```python
from build123d import *

# Parameters (mm, degrees)
F0_W     = 100
F0_H     = 270
F1_DEPTH = 100
F2_SIZE  = 75
F3_SIZE  = 5
F4_R     = 5


with BuildPart() as f1:
    # F0 (on Top) → F1 (new body)
    with BuildSketch(Plane.XY):
        Rectangle(F0_W, F0_H)
    extrude(amount=F1_DEPTH)

    # F2
    f2_edges = [f1.edges().sort_by_distance(p)[0] for p in [
        (0, -135, 0),
        (0, 135, 0),
    ]]
    chamfer(f2_edges, length=F2_SIZE)

    # F3
    f3_edges = [f1.edges().sort_by_distance(p)[0] for p in [
        (0, -135, 75),
        (0, 135, 75),
    ]]
    chamfer(f3_edges, length=F3_SIZE)

    # F4
    f4_edges = [f1.edges().sort_by_distance(p)[0] for p in [
        (0, 135, 80),
        (0, 131.464466, 71.464466),
        (0, -135, 80),
        (0, -131.464466, 71.464466),
    ]]
    fillet(f4_edges, radius=F4_R)


solid = f1.part
```
Design review of the part built by this model. Coordinates are the model's own, in mm. Give positions to 0.01 mm unless a question says otherwise; leave off trailing zeros. Loops run counter-clockwise (first coordinate to the right, second up) from the corner with the lowest first, then second, coordinate; pieces in that order, holes last. Notation, with made-up numbers: M -28.5,-25 L -17.5,-25 A36 cw -17.5,9 Z; hole C 64.5,41.25 d1. An arc over 180 degrees is marked long. Return JSON: item names as keys, results as strings. Group by question number.
Item 1: For probe 1 along Y at (x, z) = (-15, 22); probe 2 along Y at (x, z) = (-25.5, 39); probe 3 along Z at (x, y) = (5, -99.5), list the stretches that pass through material, from the lowest coordinate up.
Item 2: We need section A-A (x = 25). Give the boundary of the cut face in (y, z), and give its area (3 significant figures).
Item 3: We need section B-B (y = 108). Give the boundary of the cut face in (x, z).
Item 4: Insertion check: pin 1 Ø5 at (x, z) = (-34.5, 10) entering from +Y; pin 2 Ø4 at (x, z) = (-24.5, 16) entering from -Y; pin 3 Ø12 at (x, z) = (-12.5, 26.5) entering from -Y. Each pin has a flat end and moves straight along its axis. Give the tip position at first contact, or say it passes through.
Item 5: We need section C-C (z = 16). Give the boundary of the cut face in (x, y).
Output:
{
 "1": {"probe 1": "y = -82 to 82", "probe 2": "y = -99 to 99", "probe 3": "z = 39.5 to 100"},
 "2": {"outline": "M -135,80.99 A5 ccw -134.62,79.08 L -131.85,72.38 A5 ccw -130.76,70.76 L -60,0 L 60,0 L 130.76,70.76 A5 ccw 131.85,72.38 L 134.62,79.08 A5 ccw 135,80.99 L 135,100 L -135,100 Z", "area": "21,400 mm^2"},
 "3": {"outline": "M -50,48 L 50,48 L 50,100 L -50,100 Z"},
 "4": {"pin 1": "stops at y = 72.5", "pin 2": "stops at y = -78", "pin 3": "stops at y = -92.5"},
 "5": {"outline": "M -50,-76 L 50,-76 L 50,76 L -50,76 Z"}
}
